Here's how the part is built. I have some questions about the finished solid (model axes, mm). Give positions to 0.01 mm unless a question says otherwise; leave off trailing zeros. Loops run counter-clockwise (first coordinate to the right, second up) from the corner with the lowest first, then second, coordinate; pieces in that order, holes last.
Q1. Suppose I cut it at B-B (x = -0.45). List the corners of the cut face in (y, z) for me.
Q2. I need wall thicknesses on probe 1 along Z at (x, y) = (0.75, 0.3); probe 2 along Y at (x, z) = (-0.25, 78); probe 3 along X at (y, z) = (0.1, 219). Which ranges of each line are inside material? Lowest first, please.
Q3. Suppose I cut it at C-C (z = 72). List the corners of the cut face in (x, y) for me.
Q4. Suppose I cut it at A-A (y = 1.25). List the corners of the cut face in (x, z) for me.
```python
from build123d import *

# Parameters (mm, degrees)
CROQUIS1_R              = 2.5
SALIENTE_EXTRUIR1_DEPTH = 230
CROQUIS2_W              = 2.5
CROQUIS2_H              = 2.5
CORTAR_EXTRUIR1_DEPTH   = 5


with BuildPart() as part:
    # Croquis1 → Saliente-Extruir1 (new body)
    with BuildSketch(Plane.XY):
        Circle(CROQUIS1_R)
    extrude(amount=SALIENTE_EXTRUIR1_DEPTH)

    # Croquis2 → Cortar-Extruir1 (cut, symmetric)
    with BuildSketch(Plane(origin=(0, 0, 0), x_dir=(1, 0, 0), z_dir=(0, 1, 0))):
        with Locations((0, -115)):
            Rectangle(CROQUIS2_W, CROQUIS2_H)
    extrude(amount=CORTAR_EXTRUIR1_DEPTH, both=True, mode=Mode.SUBTRACT)


solid = part.part
```
Solutions:
1. outline: (-2.46, 0) - (2.46, 0) - (2.46, 113.75) - (-2.46, 113.75) - close; (-2.46, 116.25) - (2.46, 116.25) - (2.46, 230) - (-2.46, 230) - close
2. probe 1: z = 0 to 113.75, 116.25 to 230
2. probe 2: y = -2.49 to 2.49
2. probe 3: x = -2.5 to 2.5
3. outline: circle Ø5 at (0, 0)
4. outline: (-2.17, 0) - (2.17, 0) - (2.17, 230) - (-2.17, 230) - close; hole (-1.25, 113.75) - (1.25, 113.75) - (1.25, 116.25) - (-1.25, 116.25) - close
